from build123d import *

# Parameters (mm, degrees)
BOSS_EXTRUDE1_DEPTH     = 12
SKETCH1_3_W             = 18
SKETCH1_3_H             = 12
REVOLVE1_ANGLE          = 180
BOSS_EXTRUDE2_START     = 25
BOSS_EXTRUDE2_DEPTH     = 21
SKETCH2_W               = 34.536907577
SKETCH2_H               = 13
BOSS_EXTRUDE3_DEPTH     = 16
SKETCH3_W               = 18
SKETCH3_H               = 13
CUT_EXTRUDE2_DEPTH      = 65
BOSS_EXTRUDE4_START     = 21
SKETCH1_5_R             = 9
SKETCH1_5_R_2           = 4
BOSS_EXTRUDE4_DEPTH     = 4
CUT_EXTRUDE3_DEPTH      = 91.89004351
CUT_EXTRUDE3_DEPTH_BACK = 91.89004351
SKETCH1_6_R             = 4


with BuildPart() as part:
    # Sketch1 → Boss-Extrude1 (new body)
    with BuildSketch(Plane(origin=(0, 0, 0), x_dir=(0, 1, 0), z_dir=(0, 0, 1))):
        Polygon((31, 0), (22, 0), (22, -37), (9, -37), (9, -48), (9, -65), (-9, -65), (-9, -48), (-9, -37), (-22, -37), (-22, 0), (-31, 0), (-31, -72), (31, -72), align=None)
        Polygon((22, 37), (22, 0), (31, 0), (31, 72), (-31, 72), (-31, 0), (-22, 0), (-22, 37), (-9, 37), (-9, 48), (-9, 65), (9, 65), (9, 48), (9, 37), align=None)
        with BuildLine():
            ThreePointArc((13, 10.95445115), (15.968719423, 5.830951895), (17, 0))
            Line((17, 0), (22, 0))
            Line((22, 0), (22, 37))
            Line((22, 37), (9, 37))
            Line((9, 37), (9, 25))
            Line((9, 25), (13, 25))
            Line((13, 25), (13, 10.95445115))
        make_face()
        with BuildLine():
            Line((-22, 0), (-17, 0))
            ThreePointArc((-17, 0), (-15.968719423, 5.830951895), (-13, 10.95445115))
            Line((-13, 10.95445115), (-13, 25))
            Line((-13, 25), (-9, 25))
            Line((-9, 25), (-9, 37))
            Line((-9, 37), (-22, 37))
            Line((-22, 37), (-22, 0))
        make_face()
        with BuildLine():
            ThreePointArc((-13, -10.95445115), (-15.968719423, -5.830951895), (-17, 0))
            Line((-17, 0), (-22, 0))
            Line((-22, 0), (-22, -37))
            Line((-22, -37), (-9, -37))
            Line((-9, -37), (-9, -25))
            Line((-9, -25), (-13, -25))
            Line((-13, -25), (-13, -10.95445115))
        make_face()
        with BuildLine():
            Line((22, 0), (17, 0))
            ThreePointArc((17, 0), (15.968719423, -5.830951895), (13, -10.95445115))
            Line((13, -10.95445115), (13, -25))
            Line((13, -25), (9, -25))
            Line((9, -25), (9, -37))
            Line((9, -37), (22, -37))
            Line((22, -37), (22, 0))
        make_face()
        with BuildLine():
            Line((-13, -10.95445115), (-13, 0))
            Line((-13, 0), (-17, 0))
            ThreePointArc((-17, 0), (-15.968719423, -5.830951895), (-13, -10.95445115))
        make_face()
        with BuildLine():
            Line((-17, 0), (-13, 0))
            Line((-13, 0), (-13, 10.95445115))
            ThreePointArc((-13, 10.95445115), (-15.968719423, 5.830951895), (-17, 0))
        make_face()
        with BuildLine():
            Line((13, 10.95445115), (13, 0))
            Line((13, 0), (17, 0))
            ThreePointArc((17, 0), (15.968719423, 5.830951895), (13, 10.95445115))
        make_face()
        with BuildLine():
            Line((17, 0), (13, 0))
            Line((13, 0), (13, -10.95445115))
            ThreePointArc((13, -10.95445115), (15.968719423, -5.830951895), (17, 0))
        make_face()
    extrude(amount=-BOSS_EXTRUDE1_DEPTH)

    # Sketch1_3 → Revolve1 (revolve)
    with BuildSketch(Plane(origin=(0, 0, 0), x_dir=(0, 1, 0), z_dir=(0, 0, 1))):
        with BuildLine():
            Line((9, -25), (9, -37))
            Line((9, -37), (22, -37))
            Line((22, -37), (22, 0))
            Line((22, 0), (17, 0))
            ThreePointArc((17, 0), (15.968719423, -5.830951895), (13, -10.95445115))
            Line((13, -10.95445115), (13, -25))
            Line((13, -25), (9, -25))
        make_face()
        with Locations((0, -31)):
            Rectangle(SKETCH1_3_W, SKETCH1_3_H)
        with BuildLine():
            Line((-22, 0), (-22, -37))
            Line((-22, -37), (-9, -37))
            Line((-9, -37), (-9, -25))
            Line((-9, -25), (-13, -25))
            Line((-13, -25), (-13, -10.95445115))
            ThreePointArc((-13, -10.95445115), (-15.968719423, -5.830951895), (-17, 0))
            Line((-17, 0), (-22, 0))
        make_face()
    revolve(axis=Axis((0, -69.170626614, 0), (0, -1, 0)), revolution_arc=REVOLVE1_ANGLE)

    # Sketch1_4 → Boss-Extrude2 (add)
    with BuildSketch(Plane(origin=(0, 0, 0), x_dir=(0, 1, 0), z_dir=(0, 0, 1)).offset(BOSS_EXTRUDE2_START)):
        with BuildLine():
            ThreePointArc((-9, 0), (0, 9), (9, 0))
            Line((9, 0), (9, 14.422205102))
            ThreePointArc((9, 14.422205102), (0, 17), (-9, 14.422205102))
            Line((-9, 14.422205102), (-9, 0))
        make_face()
        with BuildLine():
            Line((9, -14.422205102), (9, 0))
            ThreePointArc((9, 0), (0, -9), (-9, 0))
            Line((-9, 0), (-9, -14.422205102))
            ThreePointArc((-9, -14.422205102), (0, -17), (9, -14.422205102))
        make_face()
        with BuildLine():
            Line((-9, -14.422205102), (-9, 0))
            Line((-9, 0), (-13, 0))
            Line((-13, 0), (-13, -10.95445115))
            ThreePointArc((-13, -10.95445115), (-11.135812919, -12.844986206), (-9, -14.422205102))
        make_face()
        with BuildLine():
            Line((-13, 0), (-9, 0))
            Line((-9, 0), (-9, 14.422205102))
            ThreePointArc((-9, 14.422205102), (-11.135812919, 12.844986206), (-13, 10.95445115))
            Line((-13, 10.95445115), (-13, 0))
        make_face()
        with BuildLine():
            Line((9, 14.422205102), (9, 0))
            Line((9, 0), (13, 0))
            Line((13, 0), (13, 10.95445115))
            ThreePointArc((13, 10.95445115), (11.135812919, 12.844986206), (9, 14.422205102))
        make_face()
        with BuildLine():
            Line((13, 0), (9, 0))
            Line((9, 0), (9, -14.422205102))
            ThreePointArc((9, -14.422205102), (11.135812919, -12.844986206), (13, -10.95445115))
            Line((13, -10.95445115), (13, 0))
        make_face()
        with BuildLine():
            Line((13, 10.95445115), (13, 0))
            Line((13, 0), (17, 0))
            ThreePointArc((17, 0), (15.968719423, 5.830951895), (13, 10.95445115))
        make_face()
        with BuildLine():
            Line((17, 0), (13, 0))
            Line((13, 0), (13, -10.95445115))
            ThreePointArc((13, -10.95445115), (15.968719423, -5.830951895), (17, 0))
        make_face()
        with BuildLine():
            Line((-13, -10.95445115), (-13, 0))
            Line((-13, 0), (-17, 0))
            ThreePointArc((-17, 0), (-15.968719423, -5.830951895), (-13, -10.95445115))
        make_face()
        with BuildLine():
            Line((-17, 0), (-13, 0))
            Line((-13, 0), (-13, 10.95445115))
            ThreePointArc((-13, 10.95445115), (-15.968719423, 5.830951895), (-17, 0))
        make_face()
    extrude(amount=BOSS_EXTRUDE2_DEPTH)

    # Sketch2 → Boss-Extrude3 (add, symmetric)
    with BuildSketch(Plane(origin=(0, 0, 0), x_dir=(-1, 0, 0), z_dir=(0, 1, 0))):
        Polygon((-65, 13), (-30.463092423, 13), (-30.463092423, 21), (-72, 21), (-72, 0), (-65, 0), align=None)
        with Locations((-47.731546212, 6.5)):
            Rectangle(SKETCH2_W, SKETCH2_H)
        with Locations((47.731546212, 6.5)):
            Rectangle(SKETCH2_W, SKETCH2_H)
        Polygon((30.463092423, 21), (30.463092423, 13), (65, 13), (65, 0), (72, 0), (72, 21), align=None)
    extrude(amount=BOSS_EXTRUDE3_DEPTH, both=True)

    # Sketch3 → Cut-Extrude2 (cut, symmetric)
    with BuildSketch(Plane.YZ):
        with Locations((0, 6.5)):
            Rectangle(SKETCH3_W, SKETCH3_H)
    extrude(amount=CUT_EXTRUDE2_DEPTH, both=True, mode=Mode.SUBTRACT)

    # Sketch1_5 → Boss-Extrude4 (add)
    # profile 1 of 2: a face of its own
    with BuildSketch(Plane(origin=(0, 0, 0), x_dir=(0, 1, 0), z_dir=(0, 0, 1)).offset(BOSS_EXTRUDE4_START)):
        with Locations(Location((0, 48, 0), (0, 0, 270))):
            Circle(SKETCH1_5_R)
        with Locations(Location((0, 48, 0), (0, 0, 270))):
            Circle(SKETCH1_5_R_2, mode=Mode.SUBTRACT)
    # profile 2 of 2: a face of its own
    with BuildSketch(Plane(origin=(0, 0, 0), x_dir=(0, 1, 0), z_dir=(0, 0, 1)).offset(BOSS_EXTRUDE4_START)):
        with Locations(Location((0, -48, 0), (0, 0, 270))):
            Circle(SKETCH1_5_R)
        with Locations(Location((0, -48, 0), (0, 0, 90))):
            Circle(SKETCH1_5_R_2, mode=Mode.SUBTRACT)
    extrude(amount=BOSS_EXTRUDE4_DEPTH)

    # Sketch1_6 → Cut-Extrude3 (cut, two sides: drawn at the far end of the back side and taken through both)
    with BuildSketch(Plane(origin=(0, 0, 0), x_dir=(0, 1, 0), z_dir=(0, 0, 1)).offset(-CUT_EXTRUDE3_DEPTH_BACK)):
        with Locations(Location((0, -48, 0), (0, 0, 270))):
            Circle(SKETCH1_6_R)
        with BuildLine():
            ThreePointArc((-9, 0), (0, -9), (9, 0))
            Line((9, 0), (-9, 0))
        make_face()
        with BuildLine():
            Line((-9, 0), (9, 0))
            ThreePointArc((9, 0), (0, 9), (-9, 0))
        make_face()
        with Locations(Location((0, 48, 0), (0, 0, 270))):
            Circle(SKETCH1_6_R)
    extrude(amount=CUT_EXTRUDE3_DEPTH + CUT_EXTRUDE3_DEPTH_BACK, mode=Mode.SUBTRACT)


solid = part.part
Here's how the part is built. I have some questions about the finished solid (model axes, mm). A direction names the side the tool comes from. Round coordinates to 2 decimals unless told otherwise and drop trailing zeros. Write each loop counter-clockwise with the first axis right and the second up, starting at its lowest first coordinate (ties: lowest second). Pieces come first, ordered by that corner, then holes.
1. Will these pins go through, and if not, where does the flat tip stop? pin 1 Ø9 at (x, y) = (-47.5, -2.5) entering from +Z; pin 2 Ø12 at (y, z) = (12, 28) entering from +X; pin 3 Ø4 at (x, z) = (10, 34.5) entering from -Y; pin 4 Ø5 at (x, y) = (-48, 0) entering from +Z.
2. Suppose I cut it at C-C (z = 7). List the corners of the cut face in (x, y) for me.
3. If we mould it in two halves opening along Y, with no side actions, what happens to faces 1 (the flat face through (-25, -11, -6)), 2 (the flat face through (-46, -4, 25)), 3 (the flat face through (1, -22, 15))? For each: released by +Y, released by -Y, zero draft, split by the parting line, or undercut.
4. Suppose I cut it at B-B (y = -6). List the corners of the cut face in (x, z) for me, and give its area (3 significant figures).
5. Suppose I cut it at D-D (y = 20). List the corners of the cut face in (x, z) for me, and give its area (3 significant figures).
6. I need wall thicknesses on L1, parallel to Y at x = -48, z = 22; L2, parallel to Y at x = -16, z = 1; L3, parallel to Z at x = 57, y = -4.5. Which ranges of each line are inside material? Lowest first, please.
7. For faces 4 (the flat face through (52, -16, 11)), 5 (the flat face through (-1, 25, 0)), 6 (the flat face through (0, 13, -1)), 7 (the flat face through (-1, -14, -12)), 8 (the cylindrical face through (-12, -14, 35)), which set-ups out of +Z, -Z, +X, -X, +Y, -Y let a thin tool reach every point of the face, with its end or its side?
8. Suppose I cut it at A-A (x = -48). List the corners of the cut face in (y, z) for me.
Answer sheet:
1. pin 1: stops at z = 25
1. pin 2: stops at x = 53.89
1. pin 3: stops at y = -22
1. pin 4: passes through
2. outline: (-72, -16) - (-36.33, -16) - (-36.33, -22) - (36.33, -22) - (36.33, -16) - (72, -16) - (72, 16) - (36.33, 16) - (36.33, 22) - (-36.33, 22) - (-36.33, 16) - (-72, 16) - close; hole (-65, -9) - (-24, -9) - (-24, -13) - (-8.43, -13) arc R15.49 ccw to (8.43, -13) - (24, -13) - (24, -9) - (65, -9) - (65, 9) - (24, 9) - (24, 13) - (8.43, 13) arc R15.49 ccw to (-8.43, 13) - (-24, 13) - (-24, 9) - (-65, 9) - close
3. face 1: undercut
3. face 2: zero draft
3. face 3: released by -Y
4. outline: (-72, -12) - (-65, -12) - (-65, 13) - (-21.35, 13) arc R25 cw to (-6.71, 24.08) - (-6.71, 46) - (-15.91, 46) - (-15.91, 33.41) arc R37 ccw to (-30.46, 21) - (-41.29, 21) - (-41.29, 25) - (-54.71, 25) - (-54.71, 21) - (-72, 21) - close; (6.71, 24.08) arc R25 cw to (21.35, 13) - (65, 13) - (65, -12) - (72, -12) - (72, 21) - (54.71, 21) - (54.71, 25) - (41.29, 25) - (41.29, 21) - (30.46, 21) arc R37 ccw to (15.91, 33.41) - (15.91, 46) - (6.71, 46) - close
4. area: 1,970 mm2
5. outline: (-72, -12) - (72, -12) - (72, 0) - (37, 0) arc R37 ccw to (-37, 0) - (-72, 0) - close
5. area: 3,880 mm2
6. L1: y = -9 to -4, 4 to 9
6. L2: y = -22 to -13, 13 to 22
6. L3: z = 13 to 21
7. face 4: +Z, +X, -Y
7. face 5: +Z, +Y
7. face 6: -Z
7. face 7: -Z, +X, -X, +Y, -Y
7. face 8: +Z
8. outline: (-31, -12) - (-9, -12) - (-9, 13) - (-4, 13) - (-4, 25) - (-9, 25) - (-9, 21) - (-16, 21) - (-16, 0) - (-31, 0) - close; (4, 13) - (9, 13) - (9, -12) - (31, -12) - (31, 0) - (16, 0) - (16, 21) - (9, 21) - (9, 25) - (4, 25) - close
